Job drawing, mm, ordinate dimensions from the low corner. One solid piece. Give positions to 0.01 mm unless a question says otherwise; leave off trailing zeros. Loops run counter-clockwise (first coordinate to the right, second up) from the corner with the lowest first, then second, coordinate; pieces in that order, holes last. Notation, with made-up numbers: (72.25, -2.5) - (83.25, -2.5) arc R24 ccw to (83.25, 28.5) - close; hole circle Ø4 at (66.25, 58.25). An arc over 180 degrees is marked (long way). Answer as CSV lines item,"result". Start each with the question number.
Item 1: Drill centre lines: L1, parallel to Z at x = 23.5, y = 7.5; L2, parallel to X at y = 5.25, z = 23; L3, parallel to Z at x = 16, y = 3. Where is each one in solid material? Low to high. Write a range as from..to.
Item 2: Saw through at B-B on x = 23.5. Give the cut face in (y, z), plus the area to 3 significant figures.
Item 3: Saw through at C-C on y = 5.5. Give the cut face in (x, z), plus the area to 3 significant figures.
Item 4: Pin check, flat tips, straight feed: pin 1 (1 mm diameter, centred on y = 7, z = 6, fed in from +X) (3 decimals); pin 2 (1.5 mm diameter, centred on x = 22.5, y = 6, fed in from +Z); pin 3 (6 mm diameter, centred on x = 18, y = 6, fed in from +Z). Stop position of each tip, or through.
Item 5: Pull direction Z, two halves, no side cores. Call the marked faces 1, 2 and 3: pulls with the +Z half, pulls with the -Z half, needs draft (parallel to the pull), parting line crosses it, or undercut.
Item 6: Saw through at A-A on z = 23.5. Give the cut face in (x, y), plus the area to 3 significant figures.
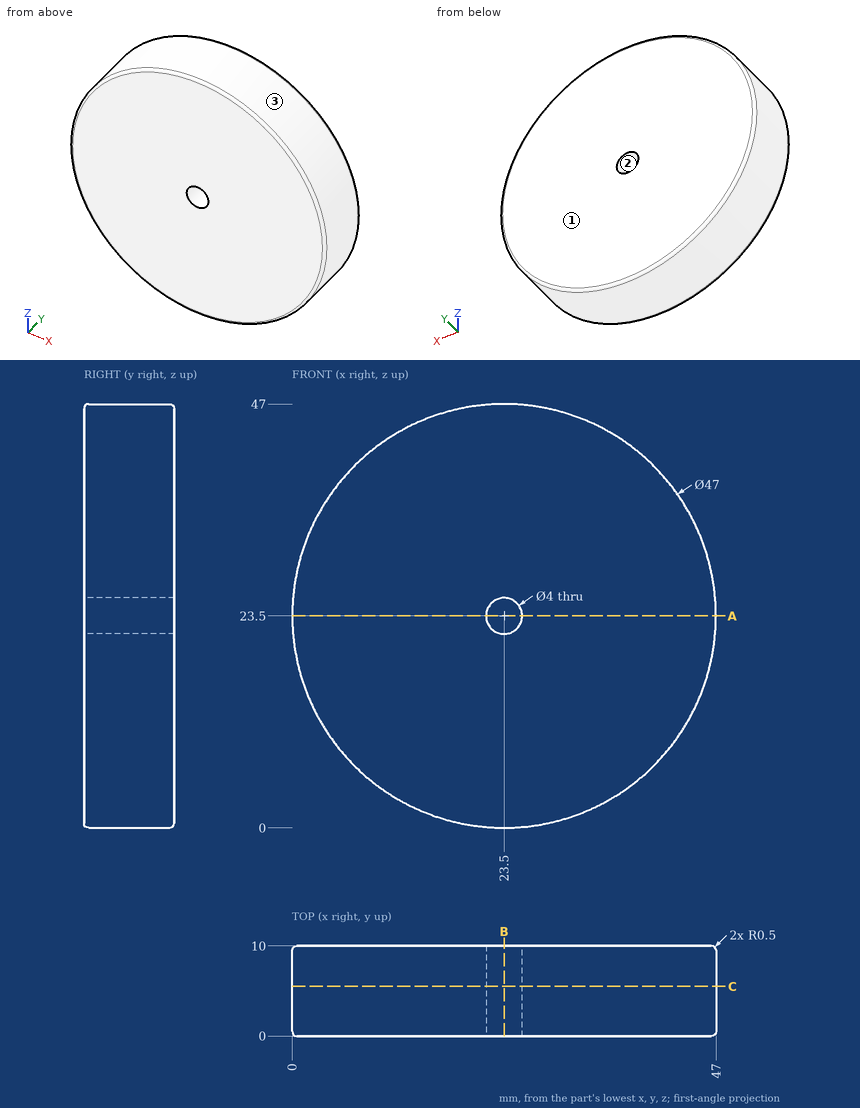
Responses:
1,L1,"0..21.5, 25.5..47"
1,L2,"0.01..21.56, 25.44..46.99"
1,L3,"1.23..45.77"
2,outline,"(0, 0.5) arc R0.5 ccw to (0.5, 0) - (9.5, 0) arc R0.5 ccw to (10, 0.5) - (10, 21.5) - (0, 21.5) - close; (0, 25.5) - (10, 25.5) - (10, 46.5) arc R0.5 ccw to (9.5, 47) - (0.5, 47) arc R0.5 ccw to (0, 46.5) - close"
2,area,"430 mm2"
3,outline,"circle Ø47 at (23.5, 23.5); hole circle Ø4 at (23.5, 23.5)"
3,area,"1,720 mm2"
4,pin 1,"x = 39.725"
4,pin 2,"z = 47"
4,pin 3,"z = 46.87"
5,face 1,"needs draft"
5,face 2,"undercut"
5,face 3,"parting line crosses it"
6,outline,"(0, 0.5) arc R0.5 ccw to (0.5, 0) - (21.5, 0) - (21.5, 10) - (0.5, 10) arc R0.5 ccw to (0, 9.5) - close; (25.5, 0) - (46.5, 0) arc R0.5 ccw to (47, 0.5) - (47, 9.5) arc R0.5 ccw to (46.5, 10) - (25.5, 10) - close"
6,area,"430 mm2"
